Can you work these out from the drawing? Everything is in mm from the part's minimum corner. A direction names the side the tool comes from. Coordinates: 2 decimals unless noted, no trailing zeros. Order: outer loops, then holes, each group sorted by start corner. A loop starts at its lowest first (then second) coordinate and runs counter-clockwise, first axis right, second up. Notation, with made-up numbers: (29, 49) - (64, 49) arc R15 cw to (64, 57) - close; hole circle Ø2 at (84, 20). An arc over 180 degrees is marked (long way). Answer as CSV lines item,"result". Start each with the question number.
Item 1: On a 3-axis mill with a long thin cutter (end or side, diameter ignored), from which of +Z, -Z, +X, -X, +Y, -Y can I reach the whole of each face in a straight line? I mean the marked faces 1 and 2. Say none if no direction works.
Item 2: I'm going to push a flat-ended pin straight in: pin 1 (4 mm diameter, centred on x = 15.875, z = 12.7, fed in from +Y) (1 decimal). Where does the tip first touch, or does it pass through?
Item 3: Imagine slicing it at B-B on z = 38.1. Count the separate pieces of the cut face and the enclosed holes in it, and give its area (3 significant figures).
Item 4: Imagine slicing it at D-D on x = 19. List the corners of the cut face in (y, z) for me (1 decimal).
Item 5: I need wall thicknesses on line 1 (X direction, y = 4, z = 38.1); line 2 (Z direction, x = 16, y = 8.75); line 3 (X direction, y = 7, z = 47) (1 decimal). Which ranges of each line are inside material? Lowest first, please.
Item 6: Imagine slicing it at A-A on x = 6.35. List the corners of the cut face in (y, z) for me (1 decimal).
Item 7: We'd pull the mould along Z, two halves only. Please class the marked faces 3, 4 and 5: pulls with the +Z half, pulls with the -Z half, needs draft (parallel to the pull), parting line crosses it, or undercut.
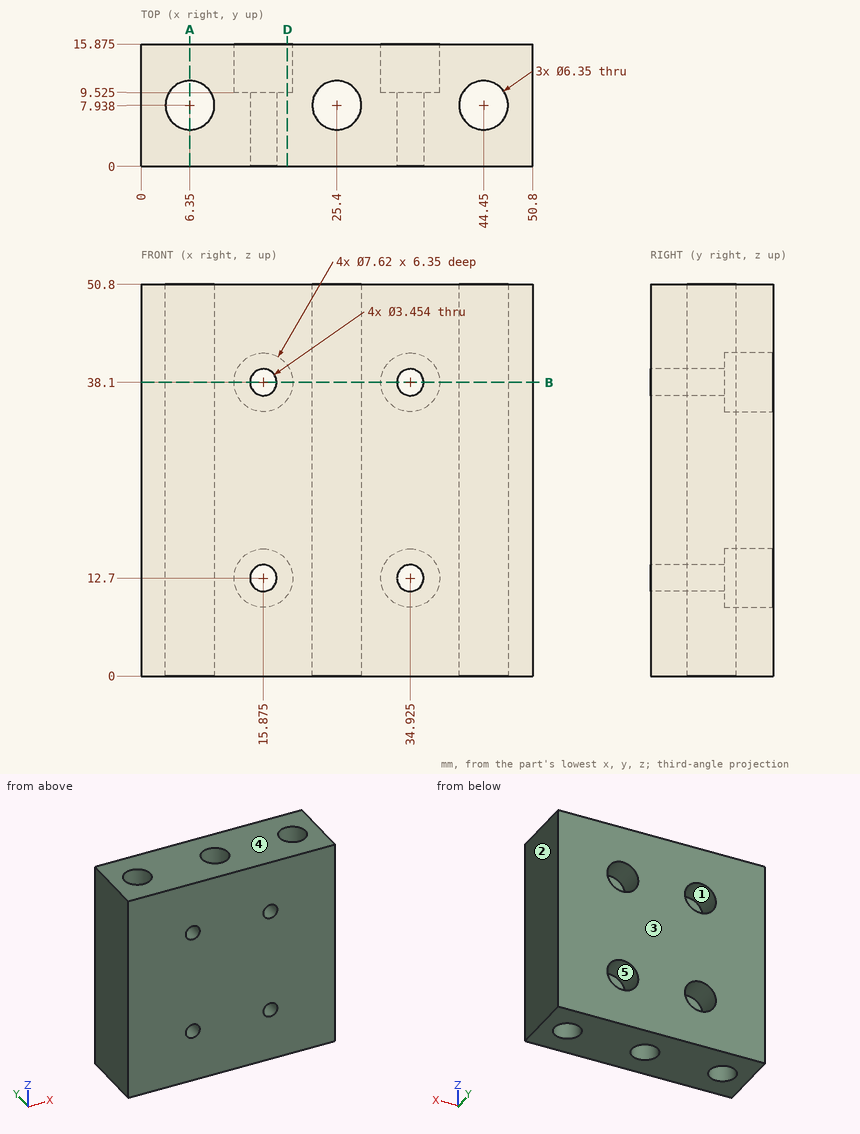
Responses:
1,face 1,"+Y"
1,face 2,"+Z, -Z, +X, +Y, -Y"
2,pin 1,"stops at y = 9.5"
3,separate pieces,"3"
3,enclosed holes,"3"
3,area,"549 mm^2"
4,outline,"(0, 0) - (15.9, 0) - (15.9, 10.5) - (9.5, 10.5) - (9.5, 14.9) - (15.9, 14.9) - (15.9, 35.9) - (9.5, 35.9) - (9.5, 40.3) - (15.9, 40.3) - (15.9, 50.8) - (0, 50.8) - close"
5,line 1,"x = 0 to 14.15, 17.6 to 33.2, 36.65 to 50.8"
5,line 2,"z = 0 to 10.98, 14.42 to 36.38, 39.82 to 50.8"
5,line 3,"x = 0 to 3.3, 9.4 to 22.4, 28.4 to 41.4, 47.5 to 50.8"
6,outline,"(0, 0) - (4.8, 0) - (4.8, 50.8) - (0, 50.8) - close; (11.1, 0) - (15.9, 0) - (15.9, 50.8) - (11.1, 50.8) - close"
7,face 3,"needs draft"
7,face 4,"pulls with the +Z half"
7,face 5,"undercut"
